```python
from build123d import *

# Parameters (mm, degrees)
ESQUISSE1_R        = 4.25
BOSS_EXTRU_1_DEPTH = 17


with BuildPart() as part:
    # Esquisse1 → Boss.-Extru.1 (new body)
    with BuildSketch(Plane(origin=(0, 0, 0), x_dir=(1, 0, 0), z_dir=(0, 1, 0))):
        Polygon((-6, 189.905239528), (0, 189.905239528), (6, 189.905239528), (16.582677371, 83.366748834), (67.130311691, 177.74566451), (72.673588887, 175.449563916), (78.216866082, 173.153463322), (52.395009204, 87.774425431), (42.899827823, 73.563882257), (31.788423162, 56.934490011), (16.702518765, 34.356838555), (-2.283322325, 38.133357153), (-7.580787473, 64.765512901), (-11.482593913, 84.381218509), (-14.816858212, 101.143697095), align=None)
        with Locations(Location((12.193145126, 61.299080025, 0), (0, 0, 270))):  # turned: the seam where the file's is
            Circle(ESQUISSE1_R, mode=Mode.SUBTRACT)
    extrude(amount=BOSS_EXTRU_1_DEPTH)


solid = part.part
```
Geometry: final body of the model. Coordinates: model frame, mm. A direction names the side the tool comes from. Coordinates: 2 decimals unless noted, no trailing zeros. Order: outer loops, then holes, each group sorted by start corner. A loop starts at its lowest first (then second) coordinate and runs counter-clockwise, first axis right, second up. Notation, with made-up numbers: (20, 68.5) -> (73, 68.5) arc R31 cw to (73, 102.5) -> close; hole circle Ø1 at (70.5, -39.75). An arc over 180 degrees is marked (long way). Write each question's results on one line, items separated by ' | '. Start each with the question number.
1) Cut plane D-D, the plane x = 1. Output: boundary loops of the cut face in (y, z), and give its area (3 significant figures).
2) Mould query, pull axis X, two halves, no side actions, for faces 3 (the flat face through (11.217, 8.381, -137.382)), 4 (the flat face through (7.34, 8.38, -36.22)), 5 (the flat face through (12, 17, -113)). Classes: released by +X, released by -X, zero draft, split by the parting line, or undercut.
3) Set-up query: faces 1 (the flat face through (0, 8, -189.905)), 2 (the flat face through (41.503, 8.381, -129.896)). Return all of +Z, -Z, +X, -X, +Y, -Y with unobstructed straight access to the full face (end or side cutting, diameter ignored); none if empty.
4) Cut plane A-A, the plane z = -167. Output: boundary loops of the cut face in (x, y).
5) First-contact query: pin 1 (6 mm diameter, centred on y = 8.5, z = -112.5, fed in from -X); pin 2 (2 mm diameter, centred on y = 4, z = -165.5, fed in from -X); pin 3 (6 mm diameter, centred on y = 6.5, z = -56, fed in from -X). Flat tips, straight axial feed; report the tip coordinate or a pass-through.
6) Material intervals for line 1 along X through (y, z) = (15.75, -121); line 2 along X through (y, z) = (15.5, -139); line 3 along X through (y, z) = (3.75, -48.5), sorted ascending.
7) Cut plane C-C, the plane z = -122.5. Output: boundary loops of the cut face in (x, y), and give its area (3 significant figures).
Checks:
1) outline: (0, -189.91) -> (17, -189.91) -> (17, -37.48) -> (0, -37.48) -> close | area: 2,590 mm^2
2) face 3: undercut | face 4: released by -X | face 5: zero draft
3) face 1: -Z, +X, -X, +Y, -Y | face 2: -Z, +Y, -Y
4) outline: (-8.28, 0) -> (8.28, 0) -> (8.28, 17) -> (-8.28, 17) -> close; (61.38, 0) -> (76.36, 0) -> (76.36, 17) -> (61.38, 17) -> close
5) pin 1: x = -13.99 | pin 2: x = -8.52 | pin 3: x = -6.43
6) line 1: -12.84 to 12.84, 36.74 to 62.44 | line 2: -11.06 to 11.06, 46.38 to 67.89 | line 3: -4.35 to 26.15
7) outline: (-12.7, 0) -> (12.7, 0) -> (12.7, 17) -> (-12.7, 17) -> close; (37.54, 0) -> (62.9, 0) -> (62.9, 17) -> (37.54, 17) -> close | area: 863 mm^2
